Build history of the part. All positions in model axes, mm. Give positions to 0.01 mm unless a question says otherwise; leave off trailing zeros. Order: outer loops, then holes, each group sorted by start corner. A loop starts at its lowest first (then second) coordinate and runs counter-clockwise, first axis right, second up. Notation, with made-up numbers: (-16.75, 10.25) - (3.25, 10.25) arc R21 ccw to (3.25, 27.25) - close; hole circle Ø2 at (34.5, 61). An arc over 180 degrees is marked (long way). Use a Markdown table: item, result.
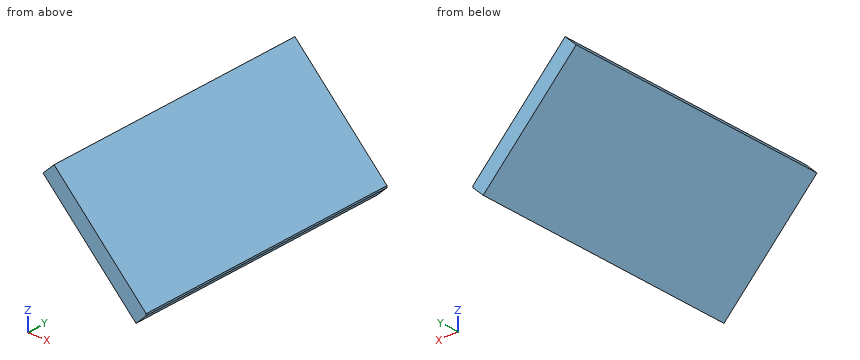
from build123d import *

# Parameters (mm, degrees)
BOX011_W               = 10
BOX011_H               = 86
BOX011_DEPTH           = 10
BOX006_W               = 5
BOX006_H               = 85
BOX006_DEPTH           = 42
BOX006_PLACEMENT_ANGLE = 315


with BuildPart() as cube011:
    # Box011 → Box011 (new body)
    with BuildSketch(Plane(origin=(55.25, 5, -33), x_dir=(1, 0, 0), z_dir=(0, 0, 1))):
        with Locations((5, 43)):
            Rectangle(BOX011_W, BOX011_H)
    extrude(amount=BOX011_DEPTH)


with BuildPart() as cut006:
    # Box006 → Box006 (new body)
    with BuildSketch(Plane.XY):
        with Locations((2.5, 42.5)):
            Rectangle(BOX006_W, BOX006_H)
    extrude(amount=BOX006_DEPTH)


with BuildPart() as cut006_1:
    # Box006 placement: moved
    add(cut006.part.moved(Location((52, 5, -33))).rotate(Axis((52, 5, -33), (0, 1, 0)), BOX006_PLACEMENT_ANGLE))

    # Cut006: cut Cube011
    add(cube011.part, mode=Mode.SUBTRACT)


solid = cut006_1.part
1) Slice it at B-B (z = -27.5). Write the cut outline in (x, y), and give its area (3 significant figures).
Computed:
| item | result |
|---|---|
| outline | (46.5, 5) - (53.57, 5) - (53.57, 90) - (46.5, 90) - close |
| area | 601 mm² |
2) Wall check: line 1 (X direction, y = 52, z = -18); line 2 (X direction, y = 51.5, z = -25.5); line 3 (Z direction, x = 27, y = 12.5). Give the ranges that are in metal, low to high. Write a range as from..to.
Computed:
| item | result |
|---|---|
| line 1 | x = 37..44.07 |
| line 2 | x = 44.5..51.57 |
| line 3 | z = -8..-0.93 |
3) Slice it at C-C (x = 51). Write the cut outline in (y, z).
Computed:
| item | result |
|---|---|
| outline | (5, -32) - (90, -32) - (90, -24.93) - (5, -24.93) - close |
4) Pin check, flat tips, straight feed: P1, Ø6, axis at x = 27, y = 15.5, coming from the +Z side; P2, Ø12, axis at y = 29.5, z = -13, coming from the +X side; P3, Ø5, axis at x = 33, y = 46, coming from the -Z side. Stop position of each tip, or through.
Computed:
| item | result |
|---|---|
| P1 | stops at z = 0.23 |
| P2 | stops at x = 45.07 |
| P3 | stops at z = -16.5 |
5) Slice it at A-A (y = 71). Write the cut outline in (x, z), and give its area (3 significant figures).
Computed:
| item | result |
|---|---|
| outline | (22.3, -3.3) - (52, -33) - (55.25, -29.75) - (55.25, -29.18) - (25.84, 0.23) - close |
| area | 210 mm² |
